from build123d import *

# Parameters (mm, degrees)
SKETCH_1_W          = 200
SKETCH_1_H          = 100
EXTRUDE_1_DEPTH     = 50
SKETCH_2_W          = 81.752741681
SKETCH_2_H          = 100
CUT_EXTRUDE_1_DEPTH = 5
SKETCH_3_W          = 93.247258319
SKETCH_3_H          = 100
CUT_EXTRUDE_2_DEPTH = 25
SKETCH_4_W          = 5
SKETCH_4_H          = 100
CUT_EXTRUDE_3_DEPTH = 20


with BuildPart() as part:
    # 草图1 → 凸台-拉伸1 (new body)
    with BuildSketch(Plane(origin=(0, 0, 0), x_dir=(1, 0, 0), z_dir=(0, 1, 0))):
        with Locations((100, 50)):
            Rectangle(SKETCH_1_W, SKETCH_1_H)
    extrude(amount=EXTRUDE_1_DEPTH)

    # 草图2 → 切除-拉伸1 (cut)
    with BuildSketch(Plane(origin=(0, 50, 0), x_dir=(1, 0, 0), z_dir=(0, 1, 0))):
        with Locations((55.876370841, 50)):
            Rectangle(SKETCH_2_W, SKETCH_2_H)
    extrude(amount=-CUT_EXTRUDE_1_DEPTH, mode=Mode.SUBTRACT)

    # 草图3 → 切除-拉伸2 (cut)
    with BuildSketch(Plane(origin=(0, 50, 0), x_dir=(1, 0, 0), z_dir=(0, 1, 0))):
        with Locations((143.37637084, 50)):
            Rectangle(SKETCH_3_W, SKETCH_3_H)
    extrude(amount=-CUT_EXTRUDE_2_DEPTH, mode=Mode.SUBTRACT)

    # 草图4 → 切除-拉伸3 (cut)
    with BuildSketch(Plane(origin=(0, 25, 0), x_dir=(1, 0, 0), z_dir=(0, 1, 0))):
        with Locations((187.5, 50)):
            Rectangle(SKETCH_4_W, SKETCH_4_H)
    extrude(amount=-CUT_EXTRUDE_3_DEPTH, mode=Mode.SUBTRACT)


solid = part.part
Input: part model. Units: mm. Frame: model coordinates. A direction names the side the tool comes from. Round coordinates to 2 decimals unless told otherwise and drop trailing zeros. Loops run counter-clockwise (first coordinate to the right, second up) from the corner with the lowest first, then second, coordinate; pieces in that order, holes last. Notation, with made-up numbers: M 77.5,19.5 L 126.5,19.5 A20 cw 126.5,40.5 Z; hole C 37,66 d3. An arc over 180 degrees is marked long. Answer as CSV lines item,"result". Start each with the question number.
(1) Section A-A, the plane y = 39.5. Output: boundary loops of the cut face in (x, z), plus the area to 3 significant figures.
(2) Section D-D, the plane x = 112. Output: boundary loops of the cut face in (y, z).
(3) First-contact query: pin 1 (12 mm diameter, centred on x = 36.5, z = -73.5, fed in from +Y); pin 2 (5.5 mm diameter, centred on x = 187, z = -43.5, fed in from +Y). Flat tips, straight axial feed; report the tip coordinate or a pass-through.
(4) Reachability of faces 4 (the flat face through (187, 5, -51)), 5 (the flat face through (76, 19, 0)) from +Z, -Z, +X, -X, +Y, -Y: full face, straight path, thin tool, end or side. Return the list, or none.
(5) Draft query along X for faces 1 (the flat face through (200, 25, -49)), 2 (the flat face through (55, 45, -51)), 3 (the flat face through (7, 50, -51)). Return one class per face: released by +X, released by -X, zero draft, split by the parting line, or undercut.
(6) Line query: line 1 (X direction, y = 21.5, z = -90.5); line 2 (X direction, y = 26, z = -49.5); line 3 (Y direction, x = 78, z = -88). Output: solid intervals per line, ascending. Write a range as [from, to].
(7) Section C-C, the plane y = 19. Output: boundary loops of the cut face in (x, z), plus the area to 3 significant figures.
(8) Section B-B, the plane z = -19. Output: boundary loops of the cut face in (x, y), plus the area to 3 significant figures.
Values found:
1,outline,"M 0,-100 L 96.75,-100 L 96.75,0 L 0,0 Z; M 190,-100 L 200,-100 L 200,0 L 190,0 Z"
1,area,"10,700 mm²"
2,outline,"M 0,-100 L 25,-100 L 25,0 L 0,0 Z"
3,pin 1,"stops at y = 45"
3,pin 2,"stops at y = 25"
4,face 4,"+Z, -Z, +Y"
4,face 5,"+Z, +X, -X, +Y, -Y"
5,face 1,"released by +X"
5,face 2,"undercut"
5,face 3,"zero draft"
6,line 1,"x = [0, 185], [190, 200]"
6,line 2,"x = [0, 96.75], [190, 200]"
6,line 3,"y = [0, 45]"
7,outline,"M 0,-100 L 185,-100 L 185,0 L 0,0 Z; M 190,-100 L 200,-100 L 200,0 L 190,0 Z"
7,area,"19,500 mm²"
8,outline,"M 0,0 L 200,0 L 200,50 L 190,50 L 190,5 L 185,5 L 185,25 L 96.75,25 L 96.75,45 L 15,45 L 15,50 L 0,50 Z"
8,area,"7,160 mm²"
